from build123d import *

# Parameters (mm, degrees)
BOX004_W          = 42
BOX004_H          = 82
BOX004_DEPTH      = 14
CYLINDER017_W     = 10
CYLINDER017_H     = 87
CYLINDER017_ANGLE = 90
CYLINDER018_R     = 15
CYLINDER018_DEPTH = 42
CYLINDER014_R     = 5.75
CYLINDER014_DEPTH = 10
CYLINDER013_R     = 3
CYLINDER013_DEPTH = 10
CYLINDER016_R     = 2
CYLINDER016_DEPTH = 94
CONE_ANGLE        = 180
CYLINDER001_W     = 10
CYLINDER001_H     = 5
CYLINDER001_ANGLE = 90
BOX002_W          = 10
BOX002_H          = 54
BOX002_DEPTH      = 11
BOX001_W          = 10
BOX001_H          = 62
BOX001_DEPTH      = 11
BOX_W             = 10
BOX_H             = 72
BOX_DEPTH         = 24
CYLINDER_W        = 10
CYLINDER_H        = 5
CYLINDER_ANGLE    = 90


with BuildPart() as include:
    # Box004 → Box004 (new body)
    with BuildSketch(Plane(origin=(-31, -36, 55), x_dir=(1, 0, 0), z_dir=(0, 0, 1))):
        with Locations((21, 41)):
            Rectangle(BOX004_W, BOX004_H)
    extrude(amount=BOX004_DEPTH)


with BuildPart() as include001:
    # Cylinder017 → Cylinder017 (revolve)
    with BuildSketch(Plane(origin=(10, -40.75, 55), x_dir=(0, 0, -1), z_dir=(1, 0, 0))):
        with Locations((5, 43.5)):
            Rectangle(CYLINDER017_W, CYLINDER017_H)
    revolve(axis=Axis((10, -40.75, 55), (0, 1, 0)), revolution_arc=CYLINDER017_ANGLE)


with BuildPart() as include002:
    # Cylinder018 → Cylinder018 (new body)
    with BuildSketch(Plane(origin=(-31, 0, 57), x_dir=(0, 1, 0), z_dir=(1, 0, 0))):
        Circle(CYLINDER018_R)
    extrude(amount=CYLINDER018_DEPTH)

    # Fusion005: union include, include001
    add(include.part)
    add(include001.part)


with BuildPart() as obj1:
    # Cylinder014 → Cylinder014 (new body)
    with BuildSketch(Plane(origin=(-23, 0, 69), x_dir=(1, 0, 0), z_dir=(0, 0, 1))):
        Circle(CYLINDER014_R)
    extrude(amount=CYLINDER014_DEPTH)


with BuildPart() as fusion003:
    # Cylinder013 → Cylinder013 (new body)
    with BuildSketch(Plane(origin=(-23, 0, 65), x_dir=(1, 0, 0), z_dir=(0, 0, 1))):
        Circle(CYLINDER013_R)
    extrude(amount=CYLINDER013_DEPTH)

    # Fusion003: union obj1
    add(obj1.part)


with BuildPart() as obj2:
    # Cylinder016 → Cylinder016 (new body)
    with BuildSketch(Plane(origin=(6, -47.35, 51), x_dir=(1, 0, 0), z_dir=(0, 1, 0))):
        Circle(CYLINDER016_R)
    extrude(amount=CYLINDER016_DEPTH)


with BuildPart() as cone:
    # Cone → Cone (revolve)
    with BuildSketch(Plane(origin=(10, 0, 65), x_dir=(0, -1, 0), z_dir=(0, 0, -1))):
        Polygon((0, 0), (15, 0), (6.5, 41), (0, 41), align=None)
    revolve(axis=Axis((10, 0, 65), (-1, 0, 0)), revolution_arc=CONE_ANGLE)


with BuildPart() as cylinder001:
    # Cylinder001 → Cylinder001 (revolve)
    with BuildSketch(Plane(origin=(10, -31, 55), x_dir=(-1, 0, 0), z_dir=(0, 0, 1))):
        with Locations((5, 2.5)):
            Rectangle(CYLINDER001_W, CYLINDER001_H)
    revolve(axis=Axis((10, -31, 55), (0, -1, 0)), revolution_arc=CYLINDER001_ANGLE)


with BuildPart() as in001:
    # Box002 → Box002 (new body)
    with BuildSketch(Plane(origin=(0, -27, 45), x_dir=(1, 0, 0), z_dir=(0, 0, 1))):
        with Locations((5, 27)):
            Rectangle(BOX002_W, BOX002_H)
    extrude(amount=BOX002_DEPTH)


with BuildPart() as in002:
    # Box001 → Box001 (new body)
    with BuildSketch(Plane(origin=(0, -31, 54), x_dir=(1, 0, 0), z_dir=(0, 0, 1))):
        with Locations((5, 31)):
            Rectangle(BOX001_W, BOX001_H)
    extrude(amount=BOX001_DEPTH)

    # Fusion: union in001
    add(in001.part)


with BuildPart() as cut:
    # Box → Box (new body)
    with BuildSketch(Plane(origin=(0, -36, 45), x_dir=(1, 0, 0), z_dir=(0, 0, 1))):
        with Locations((5, 36)):
            Rectangle(BOX_W, BOX_H)
    extrude(amount=BOX_DEPTH)

    # Cut: cut in002
    add(in002.part, mode=Mode.SUBTRACT)


with BuildPart() as common:
    # Cylinder → Cylinder (revolve)
    with BuildSketch(Plane(origin=(10, 31, 55), x_dir=(0, 0, -1), z_dir=(1, 0, 0))):
        with Locations((5, 2.5)):
            Rectangle(CYLINDER_W, CYLINDER_H)
    revolve(axis=Axis((10, 31, 55), (0, 1, 0)), revolution_arc=CYLINDER_ANGLE)

    # Fusion001: union Cylinder001, Cut
    add(cylinder001.part)
    add(cut.part)

    # Fusion004: union Cone
    add(cone.part)

    # Cut001: cut obj2
    add(obj2.part, mode=Mode.SUBTRACT)

    # Cut002: cut Fusion003
    add(fusion003.part, mode=Mode.SUBTRACT)

    # Common: intersect include002
    add(include002.part, mode=Mode.INTERSECT)


solid = common.part
Here's how the part is built. I have some questions about the finished solid (model axes, mm). A direction names the side the tool comes from. Round coordinates to 2 decimals unless told otherwise and drop trailing zeros. Order: outer loops, then holes, each group sorted by start corner. A loop starts at its lowest first (then second) coordinate and runs counter-clockwise, first axis right, second up. Notation, with made-up numbers: (45.5, 55.25) -> (85.5, 55.25) arc R29 ccw to (85.5, 82.25) -> close; hole circle Ø4 at (9.25, -33.75). An arc over 180 degrees is marked (long way). Return JSON: item names as keys, results as strings.
Q1. Which directions (+Z, -Z, +X, -X, +Y, -Y) give clear straight access to the entire face, cutting with the end or side of a thin tool? Please do faces 1 (the flat face through (5, 31, 59)), 2 (the flat face through (3, -22, 69)), 3 (the flat face through (-20.5, -2.5, 69)).
Filled sheet:
{"face 1": "+X, -X", "face 2": "+Z, +X, -X, -Y", "face 3": "+Z"}
Q2. If we section it at C-C on z = 50.25: List the corners of the cut face in (x, y) for me.
Filled sheet:
{"outline": "(1.2, -36) -> (4.15, -36) -> (4.15, -27) -> (1.2, -27) -> close; (1.2, 27) -> (4.15, 27) -> (4.15, 36) -> (1.2, 36) -> close; (7.85, -36) -> (10, -36) -> (10, -27) -> (7.85, -27) -> close; (7.85, 27) -> (10, 27) -> (10, 36) -> (7.85, 36) -> close"}
Q3. I need wall thicknesses on line 1 along X through (y, z) = (0, 67.1); line 2 along Y through (x, z) = (6, 63); line 3 along X through (y, z) = (0, 70.5). Which ranges of each line are inside material? Lowest first, please. Write a range as from..to.
Filled sheet:
{"line 1": "x = -31..-26, -20..10", "line 2": "y = -36..-31, 31..36", "line 3": "x = -31..-28.75, -17.25..10"}
Q4. If we section it at B-B on y = 0: List the corners of the cut face in (x, z) for me.
Filled sheet:
{"outline": "(-31, 65) -> (-26, 65) -> (-26, 69) -> (-28.75, 69) -> (-28.75, 71.97) -> (-31, 71.5) -> close; (-20, 65) -> (10, 65) -> (10, 72) -> (-17.25, 72) -> (-17.25, 69) -> (-20, 69) -> close"}
Q5. For pin 1 Ø1 at (x, y) = (2.5, 0.5) entering from -Z; pin 2 Ø1.5 at (y, z) = (17, 66.5) entering from -X; pin 3 Ø6 at (x, z) = (-1.5, 55.5) entering from -Y; pin 4 Ø4.5 at (x, y) = (3.5, -28) entering from +Z, each with a flat end and sliding along its axis, tell me the tip position at first contact or that it passes through.
Filled sheet:
{"pin 1": "stops at z = 65", "pin 2": "stops at x = 0", "pin 3": "stops at y = -36", "pin 4": "stops at z = 69"}
Q6. If we mould it in two halves opening along Y, with no side actions, what happens to faces 4 (the cylindrical face through (-7, 0, 72)), 5 (the flat face through (3, 23, 69)), 6 (the flat face through (5, -36, 57)), 7 (the flat face through (5, 29, 54))? For each: released by +Y, released by -Y, zero draft, split by the parting line, or undercut.
Filled sheet:
{"face 4": "split by the parting line", "face 5": "zero draft", "face 6": "released by -Y", "face 7": "undercut"}
Q7. If we section it at A-A on y = 29.5: List the corners of the cut face in (x, z) for me.
Filled sheet:
{"outline": "(0, 65) -> (10, 65) -> (10, 69) -> (0, 69) -> close; (0.05, 54) arc R10 ccw to (10, 45) -> (10, 54) -> close; hole circle Ø4 at (6, 51)"}
Q8. If we section it at D-D on x = 6: List the corners of the cut face in (y, z) for me, plus the area to 3 significant figures.
Filled sheet:
{"outline": "(-36, 45.83) -> (-27, 45.83) -> (-27, 49) -> (-36, 49) -> close; (-36, 53) -> (-27, 53) -> (-27, 54) -> (-31, 54) -> (-31, 65) -> (31, 65) -> (31, 54) -> (27, 54) -> (27, 53) -> (36, 53) -> (36, 69) -> (9, 69) arc R15 ccw to (-9, 69) -> (-36, 69) -> close; (27, 45.83) -> (36, 45.83) -> (36, 49) -> (27, 49) -> close", "area": "510 mm^2"}
